Here's how the part is built. I have some questions about the finished solid (model axes, mm). Round coordinates to 2 decimals unless told otherwise and drop trailing zeros. Write each loop counter-clockwise with the first axis right and the second up, starting at its lowest first coordinate (ties: lowest second). Pieces come first, ordered by that corner, then holes. Notation, with made-up numbers: (6.25, 6.25) -> (10.25, 6.25) arc R30 ccw to (10.25, 37.25) -> close; hole circle Ø7 at (47, 79.5). An arc over 180 degrees is marked (long way). Answer in a Markdown table with one row per item.
from build123d import *

# Parameters (mm, degrees)
SKETCH1_W           = 6.35
SKETCH1_H           = 285.75
BOSS_EXTRUDE1_DEPTH = 1.5875
CUT_EXTRUDE1_REACH  = 144.919
LPATTERN1_COUNT     = 3
LPATTERN1_PITCH     = 91.44
CUT_EXTRUDE3_DEPTH  = 2.54


with BuildPart() as part:
    # Sketch1 → Boss-Extrude1 (new body)
    with BuildSketch(Plane(origin=(0, 0, 0), x_dir=(1, 0, 0), z_dir=(0, 1, 0))):
        Rectangle(SKETCH1_W, SKETCH1_H)
    extrude(amount=BOSS_EXTRUDE1_DEPTH)

    # Sketch2 → Cut-Extrude1 (cut, up to next)
    with BuildSketch(Plane(origin=(0, 1.5875, 0), x_dir=(1, 0, 0), z_dir=(0, 1, 0)), mode=Mode.PRIVATE) as cut_extrude1_sk1:
        with BuildLine():
            Line((3.175, -139.065), (0, -139.065))
            ThreePointArc((0, -139.065), (-0.79375, -138.27125), (0, -137.4775))
            Line((0, -137.4775), (3.175, -137.4775))
            Line((3.175, -137.4775), (3.175, -139.065))
        make_face()
    cut_extrude1_tool1 = extrude(cut_extrude1_sk1.sketch, amount=-CUT_EXTRUDE1_REACH, mode=Mode.PRIVATE) & part.part
    cut_extrude1 = cut_extrude1_tool1.solids().sort_by_distance((1.271664, 1.5875, 138.27125))[0]
    add(cut_extrude1, mode=Mode.SUBTRACT)

    # LPattern1: Cut-Extrude1 ×3
    with Locations(*[(0, 0, -i * LPATTERN1_PITCH) for i in range(1, LPATTERN1_COUNT)]):
        add(cut_extrude1, mode=Mode.SUBTRACT)

    # Sketch4 → Cut-Extrude3 (cut)
    with BuildSketch(Plane(origin=(0, 1.5875, 0), x_dir=(-1, 0, 0), z_dir=(0, 1, 0))):
        with BuildLine():
            Line((-2.85454303, -136.525), (0, -136.525))
            ThreePointArc((0, -136.525), (0.79375, -135.73125), (0, -134.9375))
            Line((0, -134.9375), (-3.175, -134.9375))
            Line((-3.175, -134.9375), (-3.175, -142.875))
            Line((-3.175, -142.875), (-0.290887271, -142.875))
            Line((-0.290887271, -142.875), (-2.85454303, -136.525))
        make_face()
    extrude(amount=-CUT_EXTRUDE3_DEPTH, mode=Mode.SUBTRACT)


solid = part.part
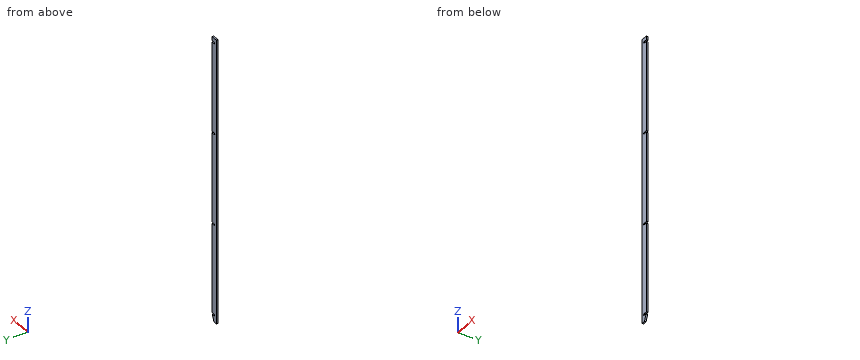
1) I want a section at B-B, the plane y = 0.95. List the corners of the cut face in (x, z) for me (1 decimal), and give its area (3 significant figures).
Response:
| item | result |
|---|---|
| outline | (-3.2, -142.9) -> (0.3, -142.9) -> (2.9, -136.5) -> (0, -136.5) arc R0.8 cw to (0, -134.9) -> (3.2, -134.9) -> (3.2, -45.4) -> (0, -45.4) arc R0.8 cw to (0, -43.8) -> (3.2, -43.8) -> (3.2, 46) -> (0, 46) arc R0.8 cw to (0, 47.6) -> (3.2, 47.6) -> (3.2, 137.5) -> (0, 137.5) arc R0.8 cw to (0, 139.1) -> (3.2, 139.1) -> (3.2, 142.9) -> (-3.2, 142.9) -> close |
| area | 1,780 mm^2 |
2) I want a section at A-A, the plane x = 1.25. List the corners of the cut face in (y, z) for me (1 decimal).
Response:
| item | result |
|---|---|
| outline | (0, -140.5) -> (1.6, -140.5) -> (1.6, -136.5) -> (0, -136.5) -> close; (0, -134.9) -> (1.6, -134.9) -> (1.6, -45.4) -> (0, -45.4) -> close; (0, -43.8) -> (1.6, -43.8) -> (1.6, 46) -> (0, 46) -> close; (0, 47.6) -> (1.6, 47.6) -> (1.6, 137.5) -> (0, 137.5) -> close; (0, 139.1) -> (1.6, 139.1) -> (1.6, 142.9) -> (0, 142.9) -> close |
3) I need wall thicknesses on line 1 (Z direction, x = -0.25, y = 0.85) (3 decimals); line 2 (Z direction, x = 0.25, y = 1.05) (1 decimal). Which ranges of each line are inside material? Lowest first, please. Write a range as [from, to].
Response:
| item | result |
|---|---|
| line 1 | z = [-142.875, -136.485], [-134.978, -45.362], [-43.855, 46.078], [47.585, 137.518], [139.025, 142.875] |
| line 2 | z = [-142.9, -136.5], [-134.9, -45.4], [-43.8, 46], [47.6, 137.5], [139.1, 142.9] |
4) For pin 1 (0.5 mm diameter, centred on x = 1, y = 1, fed in from -Z); pin 2 (0.8 mm diameter, centred on x = 1.5, y = 1, fed in from -Z), each with a flat end and sliding along its axis, tell me the tip position at first contact or that it passes through.
Response:
| item | result |
|---|---|
| pin 1 | stops at z = -141.74 |
| pin 2 | stops at z = -140.87 |
